The model under review builds one solid part; all positions refer to its coordinate system, in mm. Face numbers are marked on the shaded views. A direction names the side the tool comes from. Round coordinates to 2 decimals unless told otherwise and drop trailing zeros. Write each loop counter-clockwise with the first axis right and the second up, starting at its lowest first coordinate (ties: lowest second). Pieces come first, ordered by that corner, then holes. Notation, with made-up numbers: (9, -15.75) -> (67, -15.75) arc R10 cw to (67, -4.75) -> close; hole circle Ø5 at (16, 57). An arc over 180 degrees is marked (long way). Return JSON: item names as keys, results as strings. Group by question number.
1. Take a section at A-A, the plane z = 2.5. Write out the cut boundary in (x, y).
2. Take a section at B-B, the plane x = 13. Write out the cut boundary in (y, z), then the cut area to 3 significant figures.
3. Take a section at C-C, the plane x = 4. Write out the cut boundary in (y, z).
4. Clearance check with flat-ended pins moving along their axes: P1, Ø1.5, axis at x = -12.5, y = 16.5, coming from the -Z side; P2, Ø4, axis at y = 18.5, z = 3, coming from the +X side; P3, Ø4, axis at x = 32, z = 1.5, coming from the +Y side. State where each tip first meets the part, or that it passes through.
5. Mouldability with a two-part tool opening along Z and no side actions: class the marked faces 1, 2, 3 and 4 as pulls with the +Z half, pulls with the -Z half, needs draft (parallel to the pull), parting line crosses it, or undercut.
6. Tool access review of the marked faces 5, 6, 7 and 8: name each direction out of +Z, -Z, +X, -X, +Y, -Y from which nothing blocks a thin tool from reaching the whole face with its end or side.
7. For line 1 along Y through (x, z) = (0, 12.5); line 2 along Y through (x, z) = (30, 11.25); line 3 along X through (y, z) = (-4, -2.5), list the stretches that pass through material, from the lowest coordinate up. Write a range as from..to.
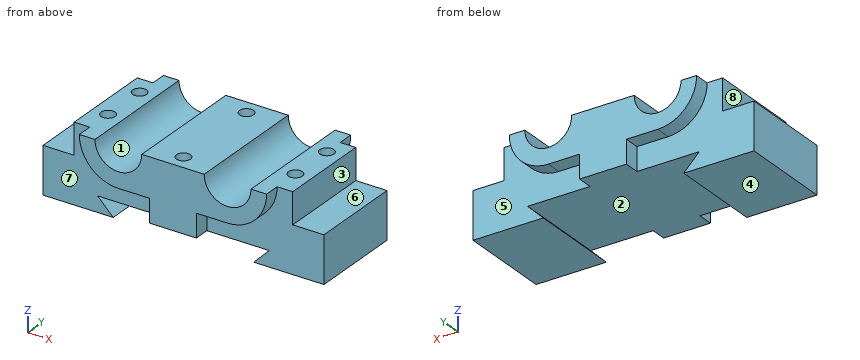
from build123d import *

# Parameters (mm, degrees)
F1_DEPTH = 15
F3_DEPTH = 5
F6_D     = 4.5
F6_DEPTH = 15
F6_TIP   = 1.3519363928


with BuildPart() as f1:
    # F0 (on Front) → F1 (new body, symmetric)
    with BuildSketch(Plane.XZ):
        with BuildLine():
            Line((-45, 10), (-45, -5))
            Line((-45, -5), (-22.5, -5))
            Line((-22.5, -5), (-27.5, 0))
            Line((-27.5, 0), (27.5, 0))
            Line((27.5, 0), (22.5, -5))
            Line((22.5, -5), (45, -5))
            Line((45, -5), (45, 10))
            Line((45, 10), (35, 10))
            Line((35, 10), (35, 20))
            Line((35, 20), (25, 20))
            ThreePointArc((25, 20), (17.5, 12.5), (10, 20))
            Line((10, 20), (-10, 20))
            ThreePointArc((-10, 20), (-17.5, 12.5), (-25, 20))
            Line((-25, 20), (-35, 20))
            Line((-35, 20), (-35, 10))
            Line((-35, 10), (-45, 10))
        make_face()
    extrude(amount=F1_DEPTH, both=True)

    # F2 (on face) → F3 (join)
    with BuildSketch(Plane.XZ.offset(15)):
        with BuildLine():
            Line((-25, 20), (-30, 20))
            ThreePointArc((-30, 20), (-26.3388347648, 11.1611652352), (-17.5, 7.5))
            Line((-17.5, 7.5), (-7.5, 7.5))
            Line((-7.5, 7.5), (-7.5, 0))
            Line((-7.5, 0), (7.5, 0))
            Line((7.5, 0), (7.5, 7.5))
            Line((7.5, 7.5), (17.5, 7.5))
            ThreePointArc((17.5, 7.5), (26.3388347648, 11.1611652352), (30, 20))
            Line((30, 20), (25, 20))
            ThreePointArc((25, 20), (17.5, 12.5), (10, 20))
            Line((10, 20), (-10, 20))
            ThreePointArc((-10, 20), (-17.5, 12.5), (-25, 20))
        make_face()
    extrude(amount=F3_DEPTH)

    # F4: F1 across plane


with BuildPart() as f1_1:
    add(f1.part)
    add(f1.part.mirror(Plane.XZ))

    # F6
    with Locations(Plane.XY.offset(20)):
        with Locations((-30, 8.6871764955), (-30, -6.3128235045), (0, 15), (0, -15), (30, 8.6871764955), (30, -6.3128235045)):
            Hole(F6_D / 2, depth=F6_DEPTH)
            with Locations((0, 0, -(F6_DEPTH + F6_TIP / 2))):  # 118° drill point
                Cone(0, F6_D / 2, F6_TIP, mode=Mode.SUBTRACT)


solid = f1_1.part
Output:
{
 "1": {"outline": "(-45, -15) -> (-7.5, -15) -> (-7.5, -20) -> (7.5, -20) -> (7.5, -15) -> (45, -15) -> (45, 15) -> (7.5, 15) -> (7.5, 20) -> (-7.5, 20) -> (-7.5, 15) -> (-45, 15) -> close"},
 "2": {"outline": "(-20, 7.5) -> (-15, 7.5) -> (-15, 0) -> (15, 0) -> (15, 7.5) -> (20, 7.5) -> (20, 14) -> (-20, 14) -> close", "area": "485 mm^2"},
 "3": {"outline": "(-20, 0) -> (20, 0) -> (20, 20) -> (-20, 20) -> close"},
 "4": {"P1": "stops at z = 7.5", "P2": "stops at x = 7.5", "P3": "stops at y = 15"},
 "5": {"face 1": "pulls with the +Z half", "face 2": "undercut", "face 3": "needs draft", "face 4": "pulls with the -Z half"},
 "6": {"face 5": "-Z, +X, +Y", "face 6": "+Z, +X, +Y, -Y", "face 7": "-Z, -X, -Y", "face 8": "+Z, -X, +Y, -Y"},
 "7": {"line 1": "y = -20..-17.25, -12.75..12.75, 17.25..20", "line 2": "y = -15..-8.56, -4.06..6.44, 10.94..15", "line 3": "x = -45..-25, 25..45"}
}
